Geometry check sheet. Reference: the model listing, model coordinates, mm. A direction names the side the tool comes from. Coordinates: 2 decimals unless noted, no trailing zeros. Order: outer loops, then holes, each group sorted by start corner. A loop starts at its lowest first (then second) coordinate and runs counter-clockwise, first axis right, second up. Notation, with made-up numbers: (72.25, 67.25) -> (80.25, 67.25) arc R15 ccw to (80.25, 76.25) -> close; hole circle Ø4 at (-8, 65.5). An arc over 180 degrees is marked (long way). Answer in a Markdown table with one row per item. Add a question column.
```python
from build123d import *

# Parameters (mm, degrees)
SKETCH_1_R               = 21
SKETCH_1_R_2             = 4
SKETCH_1_R_3             = 12.5
EXTRUDE_1_DEPTH          = 105
EXTRUDE_START            = -46
SKETCH_3_R               = 22
EXTRUDE_3_DEPTH          = 38
SKETCH_1_4_R             = 12.5
SKETCH_1_4_R_2           = 4
EXTRUDE_4_DEPTH          = 2
EXTRUDE_START_2          = -2
SKETCH_1_5_R             = 4
EXTRUDE_5_DEPTH          = 13
SKETCH_4_R               = 1.5
CUT_EXTRUDE_1_DEPTH      = 6.5
PATTERN_CIRCULAR_1_COUNT = 4


with BuildPart() as part:
    # 스케치1 → 보스-돌출1 (new body)
    # profile 1 of 3: a face of its own
    with BuildSketch(Plane.XY):
        Circle(SKETCH_1_R)
        Circle(SKETCH_1_R_2, mode=Mode.SUBTRACT)
    # profile 2 of 3: a face of its own
    with BuildSketch(Plane.XY):
        Circle(SKETCH_1_R_3)
        Circle(SKETCH_1_R_2, mode=Mode.SUBTRACT)
    # profile 3 of 3: a face of its own
    with BuildSketch(Plane.XY):
        Circle(SKETCH_1_R_2)
    extrude(amount=EXTRUDE_1_DEPTH)

    # 스케치3 → 보스-돌출3 (add)
    with BuildSketch(Plane(origin=(0, 0, 0), x_dir=(-1, 0, 0), z_dir=(0, 0, -1)).offset(EXTRUDE_START)):
        Circle(SKETCH_3_R)
    extrude(amount=-EXTRUDE_3_DEPTH)

    # 스케치1<4> → 보스-돌출4 (add)
    # profile 1 of 2: a face of its own
    with BuildSketch(Plane.XY):
        Circle(SKETCH_1_4_R)
        Circle(SKETCH_1_4_R_2, mode=Mode.SUBTRACT)
    # profile 2 of 2: a face of its own
    with BuildSketch(Plane.XY):
        Circle(SKETCH_1_4_R_2)
    extrude(amount=-EXTRUDE_4_DEPTH)

    # 스케치1<5> → 보스-돌출5 (add)
    with BuildSketch(Plane.XY.offset(EXTRUDE_START_2)):
        Circle(SKETCH_1_5_R)
    extrude(amount=-EXTRUDE_5_DEPTH)

    # 스케치4 → 컷-돌출1 (cut)
    with BuildSketch(Plane(origin=(0, 0, 0), x_dir=(-1, 0, 0), z_dir=(0, 0, -1))):
        with Locations((0, -17.5)):
            Circle(SKETCH_4_R)
    cut_extrude_1 = extrude(amount=-CUT_EXTRUDE_1_DEPTH, mode=Mode.SUBTRACT)

    # 원형 패턴1: 컷-돌출1 ×4 about axis
    pattern_circular_1_axis = Axis((0, 0, 0), (0, 0, 1))
    for i in range(1, PATTERN_CIRCULAR_1_COUNT):
        add(cut_extrude_1.rotate(pattern_circular_1_axis, i * 360 / PATTERN_CIRCULAR_1_COUNT), mode=Mode.SUBTRACT)


solid = part.part
```
(1) Go/stop test with flat-tipped pins: P1, Ø10, axis at x = -8.5, z = -1.5, coming from the +Y side; P2, Ø1, axis at x = 13.5, z = 83, coming from the +Y side; P3, Ø1.5, axis at y = -11, z = 23, coming from the -X side. Record where each tip stops, or that it passes through.
(2) Cross-section at C-C (z = 75.5). Enter the section's corners in (x, y), plus the area to 3 significant figures.
(3) Scan lines: line 1 along Y through (x, z) = (0, 2.25); line 2 along Y through (x, z) = (1, 53). Record each from-to range of solid material in increasing order.
(4) Access from +Z, -Z, +X, -X, +Y, -Y to the whole of each face (thin tool, end or side, straight path). Record for faces 1 (the face through (20.03, 6.31, 22.68)), 2 (the face through (0, 0, 105)).
(5) Mould release check, pull along Y, two halves, no side actions. Record for faces 3 (the face through (20.03, 6.31, 94.35)), 4 (the face through (0, 0, -15)), 5 (the face through (17, 0, 6.5)): +Y half, -Y half, draft (parallel to the pull), parting line (faces both ways), or undercut.
(6) Cross-section at A-A (x = -17.5). Enter the section's corners in (y, z).
(7) Cross-section at D-D (x = 0). Enter the section's corners in (y, z).
Checks:
| question | item | result |
|---|---|---|
| 1 | P1 | y = 20.67 |
| 1 | P2 | y = 17.75 |
| 1 | P3 | x = -18.33 |
| 2 | outline | circle Ø44 at (0, 0) |
| 2 | area | 1,520 mm² |
| 3 | line 1 | -21 to -19, -16 to 16, 19 to 21 |
| 3 | line 2 | -21.98 to 21.98 |
| 4 | face 1 | -Z |
| 4 | face 2 | +Z, +X, -X, +Y, -Y |
| 5 | face 3 | parting line |
| 5 | face 4 | draft |
| 5 | face 5 | undercut |
| 6 | outline | (-13.33, 46) -> (-11.61, 46) -> (-11.61, 0) -> (-1.5, 0) -> (-1.5, 6.5) -> (1.5, 6.5) -> (1.5, 0) -> (11.61, 0) -> (11.61, 46) -> (13.33, 46) -> (13.33, 84) -> (11.61, 84) -> (11.61, 105) -> (-11.61, 105) -> (-11.61, 84) -> (-13.33, 84) -> close |
| 7 | outline | (-22, 46) -> (-21, 46) -> (-21, 0) -> (-19, 0) -> (-19, 6.5) -> (-16, 6.5) -> (-16, 0) -> (-12.5, 0) -> (-12.5, -2) -> (-4, -2) -> (-4, -15) -> (4, -15) -> (4, -2) -> (12.5, -2) -> (12.5, 0) -> (16, 0) -> (16, 6.5) -> (19, 6.5) -> (19, 0) -> (21, 0) -> (21, 46) -> (22, 46) -> (22, 84) -> (21, 84) -> (21, 105) -> (-21, 105) -> (-21, 84) -> (-22, 84) -> close |
